CAD build for the part. Positions are in the model's coordinates, mm. Face numbers are marked on the shaded views. A direction names the side the tool comes from. Round coordinates to 2 decimals unless told otherwise and drop trailing zeros. Loops run counter-clockwise (first coordinate to the right, second up) from the corner with the lowest first, then second, coordinate; pieces in that order, holes last.
from build123d import *

# Parameters (mm, degrees)
CUT_EXTRUDE1_DEPTH      = 33.377264527
CUT_EXTRUDE1_DEPTH_BACK = 33.377264527
SKETCH13_R              = 3.175
CUT_EXTRUDE2_DEPTH      = 33.377264605
CUT_EXTRUDE2_DEPTH_BACK = 33.377264605
SKETCH14_W              = 12.7
SKETCH14_H              = 4.7625
CUT_EXTRUDE3_DEPTH      = 33.377264605
CUT_EXTRUDE3_DEPTH_BACK = 19.05
CUT_EXTRUDE5_START      = -3.175
CUT_EXTRUDE5_DEPTH      = 3.175
FILLET3_R               = 1.984375
CUT_EXTRUDE4_DEPTH      = 46.545358174


with BuildPart() as part:
    # Sketch1 → Revolve1 (revolve)
    with BuildSketch(Plane.XY, mode=Mode.PRIVATE) as revolve1_sk:
        Polygon((0, 26.9748), (12.6619, 26.9748), (12.6619, 22.23135), (11.43, 22.23135), (11.43, 19.84375), (12.6619, 19.84375), (12.6619, 0), (11.90625, 0), (11.90625, 11.90625), (8.73125, 11.90625), (8.73125, 23.8125), (0, 23.8125), align=None)
    revolve(revolve1_sk.sketch.rotate(Axis((0, -1015.176230553, 0), (0, 1, 0)), 90), axis=Axis((0, -1015.176230553, 0), (0, 1, 0)))

    # Sketch13 → Cut-Extrude1 (cut, two sides: drawn at the far end of the back side and taken through both)
    with BuildSketch(Plane.XY.offset(-CUT_EXTRUDE1_DEPTH_BACK)):
        with Locations((0, 15.875)):
            Circle(SKETCH13_R)
    extrude(amount=CUT_EXTRUDE1_DEPTH + CUT_EXTRUDE1_DEPTH_BACK, mode=Mode.SUBTRACT)

    # Sketch14 → Cut-Extrude2 (cut, two sides: drawn at the far end of the back side and taken through both)
    with BuildSketch(Plane.XY.offset(-CUT_EXTRUDE2_DEPTH_BACK)):
        with Locations((0, 7.14375)):
            Rectangle(SKETCH14_W, SKETCH14_H)
    extrude(amount=CUT_EXTRUDE2_DEPTH + CUT_EXTRUDE2_DEPTH_BACK, mode=Mode.SUBTRACT)

    # Sketch15 → Cut-Extrude3 (cut, two sides: drawn at the far end of the back side and taken through both)
    with BuildSketch(Plane.XZ.offset(-CUT_EXTRUDE3_DEPTH_BACK)):
        with BuildLine():
            ThreePointArc((7.9375, 8.874394786), (4.575121043, 8.687015829), (4.7625, 5.324636871))
            ThreePointArc((4.7625, 5.324636871), (7.14375, 0), (4.7625, -5.324636871))
            ThreePointArc((4.7625, -5.324636871), (4.575121043, -8.687015829), (7.9375, -8.874394786))
            ThreePointArc((7.9375, -8.874394786), (11.90625, 0), (7.9375, 8.874394786))
        make_face()
        with BuildLine():
            ThreePointArc((-4.7625, 5.324636871), (-7.14375, 0), (-4.7625, -5.324636871))
            ThreePointArc((-4.7625, -5.324636871), (-4.575121043, -8.687015829), (-7.9375, -8.874394786))
            ThreePointArc((-7.9375, -8.874394786), (-11.90625, 0), (-7.9375, 8.874394786))
            ThreePointArc((-7.9375, 8.874394786), (-4.575121043, 8.687015829), (-4.7625, 5.324636871))
        make_face()
    extrude(amount=CUT_EXTRUDE3_DEPTH + CUT_EXTRUDE3_DEPTH_BACK, mode=Mode.SUBTRACT)

    # Sketch16 → Cut-Extrude5 (cut)
    with BuildSketch(Plane(origin=(0, 26.9748, 0), x_dir=(1, 0, 0), z_dir=(0, 1, 0)).offset(CUT_EXTRUDE5_START)):
        with BuildLine():
            ThreePointArc((-8.102829044, 5.006973784), (-7.515832375, 7.303491278), (-8.34254677, 9.525))
            ThreePointArc((-8.34254677, 9.525), (-12.6619, 0), (-8.34254677, -9.525))
            ThreePointArc((-8.34254677, -9.525), (-7.515832375, -7.303491278), (-8.102829044, -5.006973784))
            ThreePointArc((-8.102829044, -5.006973784), (-9.525, 0), (-8.102829044, 5.006973784))
        make_face()
    extrude(amount=CUT_EXTRUDE5_DEPTH, mode=Mode.SUBTRACT)

    # Fillet3
    fillet3_edges = [part.edges().sort_by_distance(p)[0] for p in [
        (-7.515832375, 23.7998, 7.303491278),
        (-7.515832375, 23.7998, -7.303491278),
        (-9.525, 23.7998, 0),
    ]]
    fillet(fillet3_edges, radius=FILLET3_R)

    # 3DSketch2 → Cut-Extrude4 (cut, through all, along a direction that is not the sketch's normal)
    with BuildSketch(Plane(origin=(6.35, 26.9748, -10.954506452), x_dir=(0.2724106821506037, -0.13702750611197365, 0.9523738146436912), z_dir=(0.4493692675606063, 0.8933461039104856, 0))):
        Polygon((0, 0), (20.865570195, -6.68078041), (23.170530429, 0), (2.004022399, 6.777135294), align=None)
    extrude(amount=CUT_EXTRUDE4_DEPTH, dir=(0, 1, 0), mode=Mode.SUBTRACT)


solid = part.part
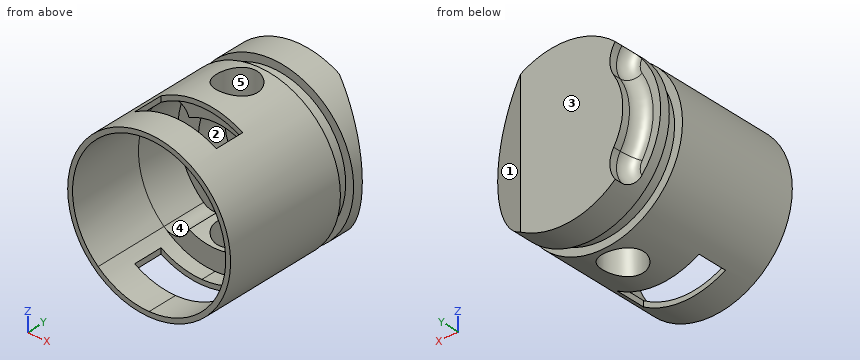
Item 1: Cut at D-D (y = 24.25). List the corners of the cut face in (x, z).
Verdict:
outline: (-8.88, -9.03) arc R12.66 ccw to (11.77, -4.68) - (11.77, 4.68) arc R12.66 ccw to (-8.88, 9.03) arc R3.24 cw to (-8.72, 5.39) arc R10.25 ccw to (-8.72, -5.39) arc R3.24 cw to start
Item 2: Cut at C-C (y = 10.5). List the corners of the cut face in (x, z).
Verdict:
outline: circle Ø25.32 at (0, 0); hole circle Ø23.81 at (0, 0)
Item 3: Mould opens along X. For the marked faces 1, 2 and 3 say: released by +X, released by -X, zero draft, split by the parting line, or undercut.
Verdict:
face 1: released by +X
face 2: undercut
face 3: zero draft
Item 4: Cut at B-B (x = 4.75). State how many separate pieces and enclosed holes the cut face has, plus the area to 3 significant figures.
Verdict:
separate pieces: 3
enclosed holes: 0
area: 163 mm2
Item 5: 3-axis set-ups, long thin cutter, end or side, ignore diameter. For the marked faces 4 and 5: which of +Z, -Z, +X, -X, +Y, -Y reach the whole face in a straight line?
Verdict:
face 4: -Y
face 5: +Z, -Z
Item 6: Flat gauge pins, fed straight in: P1, Ø8, axis at x = 6, z = 0, coming from the -Y side; P2, Ø0.8, axis at x = -3, z = 11, coming from the -Y side; P3, Ø5, axis at x = 0, y = 15.875, coming from the +Z side; P4, Ø1.5, axis at y = 4, z = -6, coming from the +X side. Where does each tip first touch, or does it go through?
Verdict:
P1: stops at y = 19.05
P2: stops at y = 11.91
P3: passes through
P4: stops at x = 11.52
Item 7: Wall check: L1, parallel to Y at x = 0, z = 9.65; L2, parallel to Y at x = 2.25, z = -3.25; L3, parallel to X at y = 16.5, z = 7.25. Give the ranges that are in metal, low to high.
Verdict:
L1: y = 11.91 to 12.7, 19.05 to 26.97
L2: y = 23.81 to 26.97
L3: x = -10.38 to -9.44, 9.44 to 10.38
